For this review, take the finished solid that the model builds, in its own axes (mm). Face numbers are marked on the shaded views. A direction names the side the tool comes from. Round coordinates to 2 decimals unless told otherwise and drop trailing zeros. Order: outer loops, then holes, each group sorted by start corner. A loop starts at its lowest first (then second) coordinate and runs counter-clockwise, first axis right, second up. Notation, with made-up numbers: M 26.5,75 L 44.5,75 A11 cw 44.5,81 Z; hole C 30.5,87.5 d2. An arc over 180 degrees is marked long. Answer as a JSON object with one key per item and string values.
from build123d import *

# Parameters (mm, degrees)
SKETCH2_R           = 4.699
SKETCH2_W           = 10.16
SKETCH2_H           = 90.4875
BOSS_EXTRUDE1_DEPTH = 9.525


with BuildPart() as part:
    # Sketch2 → Boss-Extrude1 (new body)
    with BuildSketch(Plane.XY):
        with BuildLine():
            Line((-22.220156591, -20.454196066), (-22.220156591, -149.994196066))
            Line((-22.220156591, -149.994196066), (-1.900156591, -149.994196066))
            Line((-1.900156591, -149.994196066), (-1.900156591, -20.454196066))
            ThreePointArc((-1.900156591, -20.454196066), (-12.060156591, -10.294196066), (-22.220156591, -20.454196066))
        make_face()
        with Locations(Location((-12.060156591, -21.406696066, 0), (0, 0, 180))):
            Circle(SKETCH2_R, mode=Mode.SUBTRACT)
        with Locations((-12.060156591, -99.987946066)):
            Rectangle(SKETCH2_W, SKETCH2_H, mode=Mode.SUBTRACT)
    extrude(amount=BOSS_EXTRUDE1_DEPTH)


solid = part.part
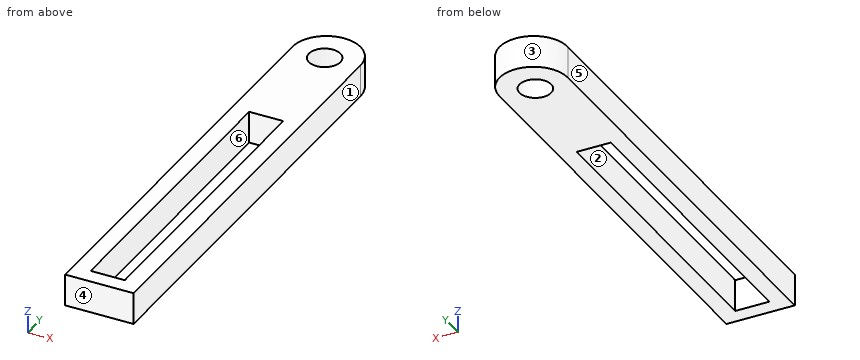
1) Mouldability with a two-part tool opening along Y and no side actions: class the marked faces 3, 4, 5 and 6 as +Y half, -Y half, draft (parallel to the pull), parting line (faces both ways), or undercut.
Geometry check:
{"face 3": "+Y half", "face 4": "-Y half", "face 5": "draft", "face 6": "undercut"}
2) For L1, parallel to X at y = -88.5, z = 2.75; L2, parallel to Y at x = -16, z = 2.75; L3, parallel to Y at x = -15, z = 7.75, list the stretches that pass through material, from the lowest coordinate up.
Geometry check:
{"L1": "x = -22.22 to -17.14, -6.98 to -1.9", "L2": "y = -149.99 to -145.23, -54.74 to -23.97, -18.85 to -11.09", "L3": "y = -149.99 to -145.23, -54.74 to -25.07, -17.74 to -10.73"}
3) Add section C-C on z = 7.5. State the section outline as (x, y) points, and give its area (3 significant figures).
Geometry check:
{"outline": "M -22.22,-149.99 L -1.9,-149.99 L -1.9,-20.45 A10.16 ccw -22.22,-20.45 Z; hole M -17.14,-145.23 L -6.98,-145.23 L -6.98,-54.74 L -17.14,-54.74 Z; hole C -12.06,-21.41 d9.4", "area": "1,810 mm²"}
4) Add section A-A on y = -66. State the section outline as (x, z) points (3 decimals), and give its area (3 significant figures).
Geometry check:
{"outline": "M -22.22,0 L -17.14,0 L -17.14,9.525 L -22.22,9.525 Z; M -6.98,0 L -1.9,0 L -1.9,9.525 L -6.98,9.525 Z", "area": "96.8 mm²"}
5) Add section B-B on x = -13.75. State the section outline as (y, z) points (3 decimals).
Geometry check:
{"outline": "M -149.994,0 L -145.232,0 L -145.232,9.525 L -149.994,9.525 Z; M -54.744,0 L -25.791,0 L -25.791,9.525 L -54.744,9.525 Z; M -17.022,0 L -10.436,0 L -10.436,9.525 L -17.022,9.525 Z"}
6) Add section D-D on x = -21. State the section outline as (y, z) points (3 decimals).
Geometry check:
{"outline": "M -149.994,0 L -15.627,0 L -15.627,9.525 L -149.994,9.525 Z"}
7) Machinability: for the marked faces 1 and 2, which of the approach directions +Z, -Z, +X, -X, +Y, -Y give a long, thin tool a straight path to every point of the face, cutting with its end or side? Answer none if there is none.
Geometry check:
{"face 1": "+Z, -Z, +X, +Y, -Y", "face 2": "+Z, -Z"}
